from build123d import *

# Parameters (mm, degrees)
BOSS_EXTRUDE1_DEPTH        = 2.54
F_8_0_199_DIAMETER_HOLE1_D = 4.191


with BuildPart() as part:
    # Sketch1 → Boss-Extrude1 (new body)
    with BuildSketch(Plane(origin=(0, 0, 0), x_dir=(1, 0, 0), z_dir=(0, 1, 0))):
        Polygon((0, 0), (0, -152.4), (107.763073453, -260.163073453), (125.723585695, -242.202561211), (25.4, 0), align=None)
    extrude(amount=BOSS_EXTRUDE1_DEPTH)

    # #8 (0.199) Diameter Hole1 (through all)
    with Locations(Plane(origin=(0, 2.54, 0), x_dir=(1, 0, 0), z_dir=(0, 1, 0))):
        with Locations((12.7, -25.4), (12.7, -50.8), (12.7, -76.2), (12.7, -101.6), (12.7, -127), (26.940768363, -161.380256121), (44.901280605, -179.340768363), (67.655118698, -202.03150109), (80.82230509, -215.261792847), (98.782817332, -233.22230509)):
            Hole(F_8_0_199_DIAMETER_HOLE1_D / 2)


solid = part.part
Source: CAD feature listing. Evaluate the final solid. Frame: model axes, mm. Coordinates: 2 decimals unless noted, no trailing zeros. Order: outer loops, then holes, each group sorted by start corner. A loop starts at its lowest first (then second) coordinate and runs counter-clockwise, first axis right, second up.
Item 1: Cut plane C-C (z = 224). Return loops of the section in (x, y), plus the area to 3 significant figures.
Output values:
outline: (71.6, 0) - (118.18, 0) - (118.18, 2.54) - (71.6, 2.54) - close
area: 118 mm2
Item 2: First-contact query: P1, Ø4, axis at x = 12.7, z = 25.4, coming from the +Y side; P2, Ø6.5, axis at x = 12.7, z = 50.8, coming from the +Y side; P3, Ø1.5, axis at x = 45, y = 1.5, coming from the -Z side. Flat tips, straight axial feed; report the tip coordinate or a pass-through.
Output values:
P1: passes through
P2: stops at y = 2.54
P3: stops at z = 45.51
Item 3: Cut plane A-A (y = 1.45). Count the separate pieces of the cut face and the enclosed holes in it, plus the area to 3 significant figures.
Output values:
separate pieces: 1
enclosed holes: 10
area: 14,500 mm2
Item 4: Cut plane B-B (x = 19). Return loops of the section in (y, z).
Output values:
outline: (0, 0) - (2.54, 0) - (2.54, 171.4) - (0, 171.4) - close
Item 5: Material intervals for line 1 (Z direction, x = 12.7, y = 1.9); line 2 (Z direction, x = 14.5, y = 1.45); line 3 (X direction, y = 1.95, z = 50.8), sorted ascending.
Output values:
line 1: z = 0 to 23.3, 27.5 to 48.7, 52.9 to 74.1, 78.3 to 99.5, 103.7 to 124.9, 129.1 to 165.1
line 2: z = 0 to 24.33, 26.47 to 49.73, 51.87 to 75.13, 77.27 to 100.53, 102.67 to 125.93, 128.07 to 166.9
line 3: x = 0 to 10.6, 14.8 to 46.44
